Design review of the part built by this model. Coordinates are the model's own, in mm. Face numbers are marked on the shaded views. A direction names the side the tool comes from. Round coordinates to 2 decimals unless told otherwise and drop trailing zeros. Loops run counter-clockwise (first coordinate to the right, second up) from the corner with the lowest first, then second, coordinate; pieces in that order, holes last. Notation, with made-up numbers: (83, 65) - (104, 65) arc R22 cw to (104, 95) - close; hole circle Ø6 at (58.5, 73). An arc over 180 degrees is marked (long way). Return JSON: item names as keys, results as strings. Group by question number.
Autodesk Inventor part; units mm, degrees
ref_plane "YZ Plane" through (0, 0, 0) normal (1, 0, 0) x (0, 1, 0)
ref_plane "XZ Plane" through (0, 0, 0) normal (0, 1, 0) x (-1, 0, 0)
ref_plane "XY Plane" through (0, 0, 0) normal (0, 0, 1) x (1, 0, 0)
sketch "Sketch1" plane through (0, 0, 0) normal (1, 0, 0) x (0, 1, 0)
  line L0 (22.0204, 19.3957) -> (-9.7296, 19.3957)
  line L1 (-9.7296, -34.5793) -> (22.0204, -34.5793)
  line L2 (22.0204, -34.5793) -> (22.0204, 19.3957)
  line L3 (15.6704, 9.8707) -> (-9.7296, 9.8707)
  line L4 (-9.7296, -25.0543) -> (15.6704, -25.0543)
  line L5 (15.6704, -25.0543) -> (15.6704, 9.8707)
  line L6 (-9.7296, 19.3957) -> (-9.7296, 9.8707)
  line L7 (-9.7296, -25.0543) -> (-9.7296, -34.5793)
  dimension "d0" = 53.975
  dimension "d2" = 6.35
  dimension "d3" = 9.525
  dimension "d4" = 9.525
  dimension "d7" = 25.4
  dimension "d8" = 0
extrude "Extrusion1" add sketch "Sketch1" along normal blind 9.525
sketch "Sketch2" plane through (0, 22.0204, 19.3957) normal (0, 1, 0) x (1, 0, 0)
  line L0 (0, 53.975) -> (9.525, 53.975)
  line L1 (0, 0) -> (9.525, 0)
  line L2 (0, 53.975) -> (0, 0)
  point P0 (0, 19.3957)
  point P1 (4.7625, 5.08)
  point P2 (4.7625, 48.895)
  dimension "d9" = 5.08
  dimension "d10" = 5.08
  dimension "d11" = 4.7625
  dimension "d12" = 0
hole "Hole1" at (4.7625, 22.0204, 14.3157) at (4.7625, 22.0204, -29.4993) direction (0, -1, 0) diameter 4.4958 end through all
sketch "Sketch4" plane through (0, 0, 0) normal (-1, 0, 0) x (0, 0, 1)
  line L0 (9.8707, 15.6704) -> (-25.0543, 15.6704)
  line L1 (9.8707, -9.7296) -> (9.8707, 15.6704)
  line L2 (-25.0543, 15.6704) -> (-25.0543, -9.7296)
  line L3 (-25.0543, 12.1144) -> (-21.4983, 15.6704)
  line L4 (-21.4983, 15.6704) -> (-25.0543, 15.6704)
  line L5 (-25.0543, 15.6704) -> (-25.0543, 12.1144)
  line L6 (9.8707, 12.1144) -> (9.8707, 15.6704)
  line L7 (9.8707, 15.6704) -> (6.3147, 15.6704)
  line L8 (6.3147, 15.6704) -> (9.8707, 12.1144)
  point P0 (0, 0)
  dimension "d20" = 45
  dimension "d21" = 3.556
  dimension "d22" = 0
  dimension "d23" = 0
  dimension "d24" = 45
  dimension "d25" = 3.556
  dimension "d26" = 0
  dimension "d27" = 0
extrude "Extrusion2" add sketch "Sketch4" against normal blind 5
sketch "Sketch5" plane through (0, 0, 0) normal (-1, 0, 0) x (0, 0, 1)
  line L0 (7.0767, 15.6704) -> (12.6647, 15.6704)
  line L1 (12.6647, 15.6704) -> (9.8707, 12.8764)
  line L2 (9.8707, 12.8764) -> (7.0767, 15.6704)
  line L3 (6.3147, 15.6704) -> (-21.4983, 15.6704)
  line L4 (-34.5793, -9.7296) -> (-34.5793, 22.0204)
  point P0 (0, 0)
  dimension "d30" = 90
  dimension "d31" = 45
  dimension "d32" = 2.794
  dimension "d33" = 0
  dimension "d34" = 44.45
extrude "Extrusion3" add sketch "Sketch5" against normal blind 5
sketch "Sketch6" plane through (0, 0, 0) normal (-1, 0, 0) x (0, 0, 1)
  line L0 (-0.2893, 9.5064) -> (-15.5293, 9.5064)
  line L1 (-15.5293, 9.5064) -> (-15.5293, 17.7024)
  line L2 (-15.5293, 17.7024) -> (-0.2893, 17.7024)
  line L3 (-0.2893, 17.7024) -> (-0.2893, 9.5064)
  line L4 (0.3457, 11.3259) -> (-14.8943, 11.3259)
  line L5 (-14.8943, 11.3259) -> (-14.8943, 17.7024)
  line L6 (-14.8943, 17.7024) -> (0.3457, 17.7024)
  line L7 (0.3457, 17.7024) -> (0.3457, 11.3259)
  line L8 (6.3147, 15.6704) -> (-21.4983, 15.6704)
  line L9 (-34.5793, -9.7296) -> (-34.5793, 22.0204)
  line L10 (19.3957, 22.0204) -> (19.3957, -9.7296)
  point P0 (0, 0)
  point P1 (12.6647, 15.6704)
  dimension "d37" = 2.032
  dimension "d38" = 0
  dimension "d39" = 19.05
  dimension "d40" = 19.05
  dimension "d42" = 15.24
  dimension "d43" = 15.24
extrude "Extrusion4" cut sketch "Sketch6" against normal blind 254
properties part number "OneSparkMaxTop"
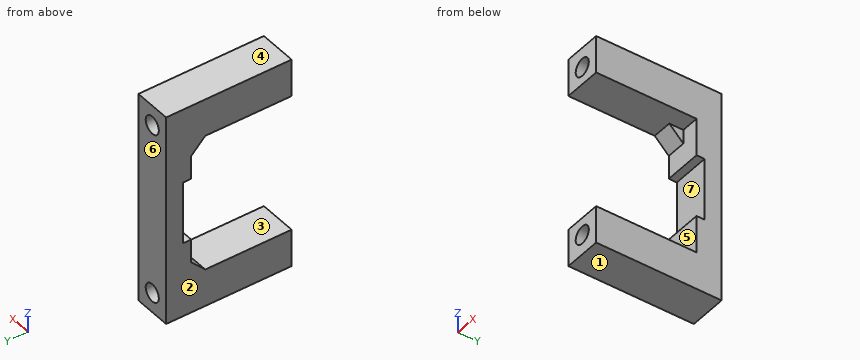
Q1. Add section D-D, the plane x = 1.25. State the section outline as (y, z) points.
Q2. Tool access review of the marked faces 5, 6 and 7: name each direction out of +Z, -Z, +X, -X, +Y, -Y from which nothing blocks a thin tool from reaching the whole face with its end or side.
Q3. Add section C-C, the plane x = 4. State the section outline as (y, z) points, plus the area to 3 significant figures.
Q4. Add section A-A, the plane y = 6.5. State the section outline as (x, z) points (1 decimal).
Q5. For line 1 (Z direction, x = 2, y = 8); line 2 (Z direction, x = 9, y = 16); line 3 (Z direction, x = 3, y = 0.5), list the stretches that pass through material, from the lowest coordinate up.
Q6. Add section B-B, the plane z = -28. State the section outline as (x, y) points (3 decimals), plus the area to 3 significant figures.
Q7. Insertion check: pin 1 Ø5 at (x, z) = (5.5, -11) entering from -Y; pin 2 Ø3 at (x, z) = (7, -18) entering from -Y; pin 3 Ø4 at (y, z) = (14.5, -22.5) entering from +X (3 decimals); pin 4 Ø1.1 at (y, z) = (14, 7.5) entering from +X. Each pin has a flat end and moves straight along its axis. Give the tip position at first contact, or say it passes through.
Q8. Draft analysis for pull direction Z (two halves, no side actions). For the marked faces 1, 2, 3 and 4, state which applies: pulls with the +Z half, pulls with the -Z half, needs draft (parallel to the pull), parting line crosses it, or undercut.
Evaluation:
{
 "1": {"outline": "(-9.73, -34.58) - (22.02, -34.58) - (22.02, 19.4) - (-9.73, 19.4) - (-9.73, 9.87) - (12.11, 9.87) - (15.67, 6.31) - (15.67, 0.35) - (17.7, 0.35) - (17.7, -15.53) - (15.67, -15.53) - (15.67, -21.5) - (12.11, -25.05) - (-9.73, -25.05) - close"},
 "2": {"face 5": "+X, -Y", "face 6": "+Z, -Z, +X, -X, +Y", "face 7": "+X, -X, -Y"},
 "3": {"outline": "(-9.73, -34.58) - (22.02, -34.58) - (22.02, -31.61) - (-9.73, -31.61) - close; (-9.73, -27.38) - (22.02, -27.38) - (22.02, 12.2) - (15.67, 12.2) - (15.67, 12.66) - (15.21, 12.2) - (-9.73, 12.2) - (-9.73, 9.87) - (12.11, 9.87) - (15.67, 6.31) - (15.67, 0.35) - (17.7, 0.35) - (17.7, -15.53) - (15.67, -15.53) - (15.67, -21.5) - (12.11, -25.05) - (-9.73, -25.05) - close; (-9.73, 16.43) - (22.02, 16.43) - (22.02, 19.4) - (-9.73, 19.4) - close", "area": "539 mm²"},
 "4": {"outline": "(0, -34.6) - (9.5, -34.6) - (9.5, -25.1) - (0, -25.1) - close; (0, 9.9) - (9.5, 9.9) - (9.5, 19.4) - (0, 19.4) - close; hole circle Ø4.5 at (4.8, -29.5); hole circle Ø4.5 at (4.8, 14.3)"},
 "5": {"line 1": "-34.58 to -25.05, 9.87 to 19.4", "line 2": "-34.58 to -15.53, 0.35 to 19.4", "line 3": "-34.58 to -30.89, -28.1 to -25.05, 9.87 to 12.92, 15.71 to 19.4"},
 "6": {"outline": "(0, -9.73) - (3.088, -9.73) - (3.088, 22.02) - (0, 22.02) - close; (6.437, -9.73) - (9.525, -9.73) - (9.525, 22.02) - (6.437, 22.02) - close", "area": "196 mm²"},
 "7": {"pin 1": "y = 17.7", "pin 2": "y = 15.67", "pin 3": "x = 9.525", "pin 4": "x = 5"},
 "8": {"face 1": "pulls with the -Z half", "face 2": "needs draft", "face 3": "undercut", "face 4": "pulls with the +Z half"}
}
